Check sheet for the drawn part. Datum: minimum x, y, z corner. Units: mm. Give positions to 0.01 mm unless a question says otherwise; leave off trailing zeros. Order: outer loops, then holes, each group sorted by start corner. A loop starts at its lowest first (then second) coordinate and runs counter-clockwise, first axis right, second up. Notation, with made-up numbers: M -3,-22 L 47,-22 A17 cw 47,-8 Z; hole C 12,39.25 d4. An arc over 180 degrees is marked long. Answer as CSV lines item,"result". Start each with the question number.
Q1. Go/stop test with flat-tipped pins: pin 1 (6 mm diameter, centred on x = 813, z = 8, fed in from +Y); pin 2 (8 mm diameter, centred on y = 194.5, z = 16.5, fed in from -X). Record where each tip stops, or that it passes through.
Q2. Section check C-C, the plane x = 757.5. Record the boundary of the cut face in (y, z).
Q3. Section check D-D, the plane x = 359.5. Record the boundary of the cut face in (y, z).
Q4. Thickness scan on line 1 (Y direction, x = 945, z = 12); line 2 (X direction, y = 155, z = 3) (1 decimal); line 3 (Y direction, x = 850, z = 13.75). Record the ranges inside material, lowest first.
Q5. Section check B-B, the plane y = 150. Record the boundary of the cut face in (x, z) (3 decimals).
Q6. Section check A-A, the plane z = 4.25. Record the boundary of the cut face in (x, y) (3 decimals).
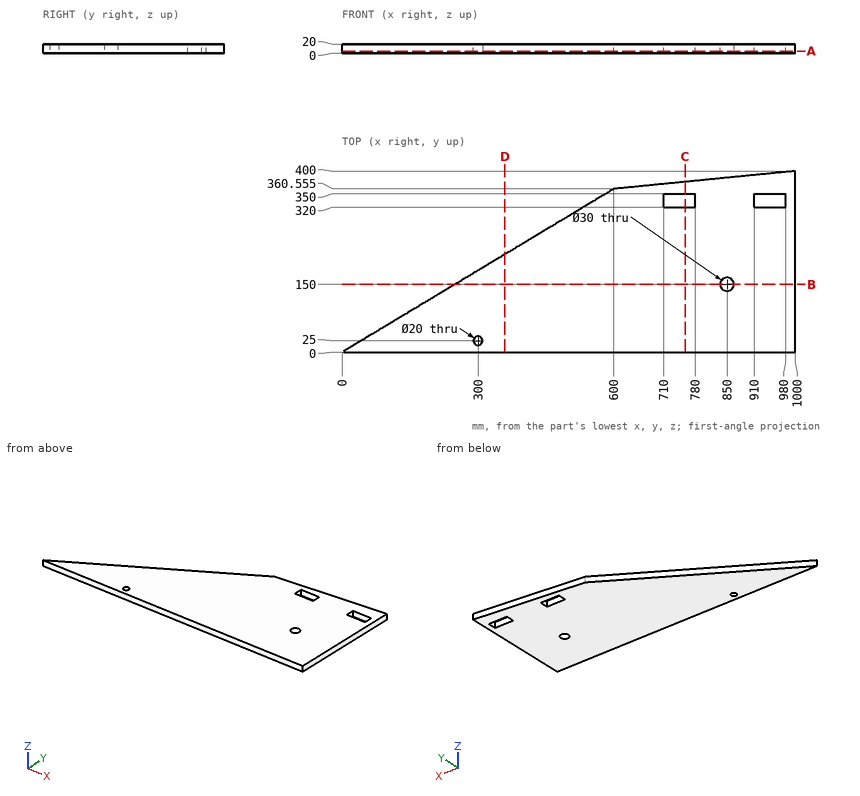
Answer block:
1,pin 1,"stops at y = 381.86"
1,pin 2,"stops at x = 317.01"
2,outline,"M 0,0 L 320,0 L 320,20 L 0,20 Z; M 350,0 L 376.09,0 L 376.09,20 L 350,20 Z"
3,outline,"M 0,0 L 216.03,0 L 216.03,20 L 0,20 Z"
4,line 1,"y = 0 to 320, 350 to 394.58"
4,line 2,"x = 257.9 to 835.9, 864.1 to 1000"
4,line 3,"y = 0 to 135, 165 to 385.21"
5,outline,"M 249.615,0 L 835,0 L 835,20 L 249.615,20 Z; M 865,0 L 1000,0 L 1000,20 L 865,20 Z"
6,outline,"M 0,0 L 1000,0 L 1000,400 L 600,360.555 Z; hole C 300,25 d20; hole M 710,320 L 780,320 L 780,350 L 710,350 Z; hole C 850,150 d30; hole M 910,320 L 980,320 L 980,350 L 910,350 Z"
